Design review of the part built by this model. Coordinates are the model's own, in mm. A direction names the side the tool comes from. Coordinates: 2 decimals unless noted, no trailing zeros. Loops run counter-clockwise (first coordinate to the right, second up) from the corner with the lowest first, then second, coordinate; pieces in that order, holes last. Notation, with made-up numbers: (70, 23.25) -> (75, 23.25) arc R32 cw to (75, 55.25) -> close; hole circle Ø11 at (-32.75, 52.25). An arc over 180 degrees is marked (long way). Use a Markdown table: item, result. Add a question column.
Q1. Clearance check with flat-ended pins moving along their axes: pin 1 Ø12 at (x, y) = (17.5, 44) entering from -Z; pin 2 Ø16.5 at (x, y) = (-0.5, -3) entering from +Z; pin 3 Ø1.5 at (x, z) = (-3, -26.5) entering from +Y; pin 4 Ø19 at (x, y) = (-8, 99) entering from +Z. State where each tip first meets the part, or that it passes through.
Q2. Take a section at D-D on z = -38. Write out the cut boundary in (x, y), plus the area to 3 significant figures.
Q3. Draft analysis for pull direction X (two halves, no side actions). For faces 1 (the face through (-2.47, 108.84, -30.21)), 2 (the face through (-14, 14, -45)), 3 (the face through (-1.302, 99.915, -30.21)), state which applies: pulls with the +X half, pulls with the -X half, needs draft (parallel to the pull), parting line crosses it, or undercut.
Q4. For faces 4 (the face through (8, 82, -15)), 5 (the face through (8, 82, -45)), 6 (the face through (14, -24, -15)), list the 3-axis set-ups (+Z, -Z, +X, -X, +Y, -Y) from which the entire face can be reached by the end or side of a thin tool; tool diameter is ignored.
Q5. For probe 1 along Y at (x, z) = (0, -33); probe 2 along Z at (x, y) = (4.5, 52); probe 3 along Z at (x, y) = (10.5, 28), list the stretches that pass through material, from the lowest coordinate up.
Q6. Take a section at C-C on z = -17. Write out the cut boundary in (x, y), plus the area to 3 significant figures.
Q7. Take a section at B-B on y = 90. Write out the cut boundary in (x, z), plus the area to 3 significant figures.
Q8. Take a section at A-A on x = 0. Write out the cut boundary in (y, z).
from build123d import *

# Parameters (mm, degrees)
SKETCH2_R                = 27.5
SKETCH2_R_2              = 21.5
CUT_EXTRUDE1_DEPTH       = 5
BOSS_EXTRUDE1_DEPTH      = 15
BOSS_EXTRUDE1_DEPTH_BACK = 15
SKETCH3_R                = 19
SKETCH3_R_2              = 10
BOSS_EXTRUDE2_DEPTH      = 5
BOSS_EXTRUDE2_DEPTH_BACK = 5


with BuildPart() as part:
    # Sketch1 → Revolve1 (revolve)
    with BuildSketch(Plane(origin=(0, 0, 0), x_dir=(0, 0, -1), z_dir=(1, 0, 0)), mode=Mode.PRIVATE) as revolve1_sk:
        Polygon((0, 17), (45, 17), (45, 32), (15, 32), (15, 21.5), (0, 21.5), align=None)
    revolve(revolve1_sk.sketch.rotate(Axis((0, 0, 0), (0, 0, -1)), 90), axis=Axis((0, 0, 0), (0, 0, -1)))

    # Sketch2 → Cut-Extrude1 (cut)
    with BuildSketch(Plane.XY.offset(-15)):
        Circle(SKETCH2_R)
        Circle(SKETCH2_R_2, mode=Mode.SUBTRACT)
    extrude(amount=-CUT_EXTRUDE1_DEPTH, mode=Mode.SUBTRACT)



with BuildPart() as body_2:
    # Sketch3 → Boss-Extrude1 (new, two sides: drawn at the far end of the back side and taken through both)
    with BuildSketch(Plane.XY.offset(-30).offset(-BOSS_EXTRUDE1_DEPTH_BACK)):
        with Locations((0, 90)):
            Circle(SKETCH3_R)
        with Locations((0, 90)):
            Circle(SKETCH3_R_2, mode=Mode.SUBTRACT)
    extrude(amount=BOSS_EXTRUDE1_DEPTH + BOSS_EXTRUDE1_DEPTH_BACK)


with BuildPart() as part_1:
    add(part.part)

    add(body_2.part)  # Boss-Extrude2 merges body 2
    # Sketch4 → Boss-Extrude2 (add, two sides: drawn at the far end of the back side and taken through both)
    with BuildSketch(Plane.XY.offset(-30).offset(-BOSS_EXTRUDE2_DEPTH_BACK)):
        with BuildLine():
            ThreePointArc((25.517690077, 19.309259259), (0, 32), (-25.517690077, 19.309259259))
            ThreePointArc((-25.517690077, 19.309259259), (-13.056566583, 49.915660424), (-17.5241968, 82.658165997))
            ThreePointArc((-17.5241968, 82.658165997), (0, 71), (17.5241968, 82.658165997))
            ThreePointArc((17.5241968, 82.658165997), (13.056566583, 49.915660424), (25.517690077, 19.309259259))
        make_face()
    extrude(amount=BOSS_EXTRUDE2_DEPTH + BOSS_EXTRUDE2_DEPTH_BACK)


solid = part_1.part
Answer list:
| question | item | result |
|---|---|---|
| 1 | pin 1 | z = -35 |
| 1 | pin 2 | through |
| 1 | pin 3 | y = 108.87 |
| 1 | pin 4 | z = -15 |
| 2 | outline | circle Ø64 at (0, 0); circle Ø38 at (0, 90); hole circle Ø34 at (0, 0); hole circle Ø20 at (0, 90) |
| 2 | area | 3,130 mm² |
| 3 | face 1 | parting line crosses it |
| 3 | face 2 | needs draft |
| 3 | face 3 | undercut |
| 4 | face 4 | +Z, +X, -X, +Y |
| 4 | face 5 | -Z, +X, -X, +Y, -Y |
| 4 | face 6 | +Z |
| 5 | probe 1 | -32 to -17, 17 to 80, 100 to 109 |
| 5 | probe 2 | -35 to -25 |
| 5 | probe 3 | -45 to -15 |
| 6 | outline | circle Ø64 at (0, 0); circle Ø43 at (0, 0); circle Ø38 at (0, 90); hole circle Ø55 at (0, 0); hole circle Ø34 at (0, 0); hole circle Ø20 at (0, 90) |
| 6 | area | 2,210 mm² |
| 7 | outline | (-19, -45) -> (-10, -45) -> (-10, -15) -> (-19, -15) -> close; (10, -45) -> (19, -45) -> (19, -15) -> (10, -15) -> close |
| 7 | area | 540 mm² |
| 8 | outline | (-32, -45) -> (-17, -45) -> (-17, 0) -> (-21.5, 0) -> (-21.5, -20) -> (-27.5, -20) -> (-27.5, -15) -> (-32, -15) -> close; (17, -45) -> (32, -45) -> (32, -35) -> (71, -35) -> (71, -45) -> (80, -45) -> (80, -15) -> (71, -15) -> (71, -25) -> (32, -25) -> (32, -15) -> (27.5, -15) -> (27.5, -20) -> (21.5, -20) -> (21.5, 0) -> (17, 0) -> close; (100, -45) -> (109, -45) -> (109, -15) -> (100, -15) -> close |
